Check sheet for the modelled part. Datum: model origin and axes. Units: mm. A direction names the side the tool comes from. Give positions to 0.01 mm unless a question says otherwise; leave off trailing zeros. Order: outer loops, then holes, each group sorted by start corner. A loop starts at its lowest first (then second) coordinate and runs counter-clockwise, first axis right, second up.
Item 1: Sectioned sample at A-A on y = 71.5. Record the boundary of the cut face in (x, z), and give its area (3 significant figures).
Item 2: Sectioned sample at B-B on z = 7.5. Count the separate pieces of the cut face and the enclosed holes in it, and give its area (3 significant figures).
Item 3: Access from +Z, -Z, +X, -X, +Y, -Y to the whole of each face (thin tool, end or side, straight path). Record for faces 4 (the flat face through (288, 169, 12.395)), 5 (the flat face through (408, 0, 6)), 6 (the flat face through (187.78, 223.79, 6.11)), 7 (the flat face through (409.074, 70, 6)), 8 (the flat face through (565, 0, 6)).
Item 4: Sectioned sample at C-C on x = 95.5. Record the boundary of the cut face in (y, z), and give its area (3 significant figures).
Item 5: Sectioned sample at D-D on y = 290.5. Record the boundary of the cut face in (x, z), and give its area (3 significant figures).
Item 6: Release check for a two-part mould opening along X. For faces 1 (the flat face through (421.47, 70, 6)), 2 (the flat face through (478.786, 217.611, 6.111)), 3 (the flat face through (19, 0, 6)) record: released by +X, released by -X, zero draft, split by the parting line, or undercut.
Item 7: Gauge pin test, flat ends, axial feed: P1, Ø6, axis at x = 16.5, z = 6, coming from the -Y side; P2, Ø6, axis at y = 71, z = 8.5, coming from the +X side; P3, Ø3.5, axis at y = 71, z = 6, coming from the +X side. Record the tip position at first contact, or that the pin passes through.
Item 8: Material ranges on line 1 along X through (y, z) = (65, 8.75); line 2 along X through (y, z) = (88, 8); line 3 along Y through (x, z) = (331, 3.5), recorded low to high.
from build123d import *

# Parameters (mm, degrees)
F1_DEPTH = 12.3952
F2_W     = 38.1
F2_H     = 12.3952
F3_DEPTH = 9.2964
F4_W     = 12.3952
F4_H     = 38.1
F5_DEPTH = 12.3952


with BuildPart() as f1:
    # F0 (on Top) → F1 (new body)
    with BuildSketch(Plane.XY):
        with BuildLine():
            Line((370.379511, 441.401113), (0, 0))
            Line((0, 0), (370.379511, 0))
            Line((370.379511, 0), (370.379511, 88.52408))
            ThreePointArc((370.379511, 88.52408), (359.660711, 99.24288), (370.379511, 109.96168))
            Line((370.379511, 109.96168), (370.379511, 203.119918))
            ThreePointArc((370.379511, 203.119918), (359.660711, 213.838718), (370.379511, 224.557518))
            Line((370.379511, 224.557518), (370.379511, 359.660723))
            ThreePointArc((370.379511, 359.660723), (359.660711, 370.379523), (370.379511, 381.098323))
            Line((370.379511, 381.098323), (370.379511, 441.401113))
        make_face()
        with BuildLine():
            Line((370.379511, 88.52408), (370.379511, 0))
            Line((370.379511, 0), (584.2, 0))
            Line((584.2, 0), (370.379511, 441.401113))
            Line((370.379511, 441.401113), (370.379511, 381.098323))
            ThreePointArc((370.379511, 381.098323), (377.958847, 377.95886), (381.098311, 370.379523))
            ThreePointArc((381.098311, 370.379523), (377.958847, 362.800187), (370.379511, 359.660723))
            Line((370.379511, 359.660723), (370.379511, 224.557518))
            ThreePointArc((370.379511, 224.557518), (377.958847, 221.418054), (381.098311, 213.838718))
            ThreePointArc((381.098311, 213.838718), (377.958847, 206.259381), (370.379511, 203.119918))
            Line((370.379511, 203.119918), (370.379511, 109.96168))
            ThreePointArc((370.379511, 109.96168), (377.958847, 106.822216), (381.098311, 99.24288))
            ThreePointArc((381.098311, 99.24288), (377.958847, 91.663544), (370.379511, 88.52408))
        make_face()
    extrude(amount=F1_DEPTH)

    # F2 (on face) → F3 (join)
    with BuildSketch(Plane.XZ):
        with Locations((57.15, 6.1976)):
            Rectangle(F2_W, F2_H)
        with Locations((292.1, 6.1976)):
            Rectangle(F2_W, F2_H)
        with Locations((527.05, 6.1976)):
            Rectangle(F2_W, F2_H)
    extrude(amount=F3_DEPTH)

    # F4 (on face) → F5 (cut, through all)
    with BuildSketch(Plane.XY.offset(12.3952)):
        with Locations((238.691288, 70.7644)):
            Rectangle(F4_W, F4_H)
        with Locations((326.981688, 70.7644)):
            Rectangle(F4_W, F4_H)
        with Locations((415.272088, 70.7644)):
            Rectangle(F4_W, F4_H)
        with Locations((175.800888, 70.7644)):
            Rectangle(F4_W, F4_H)
    extrude(amount=-F5_DEPTH, mode=Mode.SUBTRACT)


solid = f1.part
Report:
1. outline: (60, 0) - (169.6, 0) - (169.6, 12.4) - (60, 12.4) - close; (182, 0) - (232.49, 0) - (232.49, 12.4) - (182, 12.4) - close; (244.89, 0) - (320.78, 0) - (320.78, 12.4) - (244.89, 12.4) - close; (333.18, 0) - (409.07, 0) - (409.07, 12.4) - (333.18, 12.4) - close; (421.47, 0) - (549.56, 0) - (549.56, 12.4) - (421.47, 12.4) - close
1. area: 5,450 mm2
2. separate pieces: 1
2. enclosed holes: 7
2. area: 127,000 mm2
3. face 4: +Z, +X, -X, +Y, -Y
3. face 5: +Z, -Z, -Y
3. face 6: +Z, -Z, -X, +Y
3. face 7: +Z, -Z
3. face 8: +Z, -Z, +X, -Y
4. outline: (0, 0) - (113.81, 0) - (113.81, 12.4) - (0, 12.4) - close
4. area: 1,410 mm2
5. outline: (243.76, 0) - (443.48, 0) - (443.48, 12.4) - (243.76, 12.4) - close
5. area: 2,480 mm2
6. face 1: undercut
6. face 2: released by +X
6. face 3: zero draft
7. P1: stops at y = 0
7. P2: stops at x = 551.26
7. P3: stops at x = 550.65
8. line 1: x = 54.54 to 169.6, 182 to 232.49, 244.89 to 320.78, 333.18 to 409.07, 421.47 to 552.71
8. line 2: x = 73.84 to 169.6, 182 to 232.49, 244.89 to 320.78, 333.18 to 409.07, 421.47 to 541.57
8. line 3: y = 0 to 51.71, 89.81 to 394.47
